Verification items for the finished model (mm, model axes). Coordinates: 2 decimals unless noted, no trailing zeros. Loops run counter-clockwise (first coordinate to the right, second up) from the corner with the lowest first, then second, coordinate; pieces in that order, holes last. Notation, with made-up numbers: (74, -35) - (131, -35) arc R30 ccw to (131, 0) - close; hole circle Ø7 at (-27, -6). An arc over 180 degrees is marked (long way). One line per item, written item: value. Start each with the question number.
(1) Gauge pin test, flat end, axial feed: P1, Ø1.5, axis at x = 122, y = 0.5, coming from the +Z side. Record the tip position at first contact, or that the pin passes through.
(2) Thickness scan on probe 1 along X at (y, z) = (0.95, 63); probe 2 along Z at (x, y) = (77, 2.3). Record the ranges inside material, lowest first. Write a range as [from, to].
(3) Section check B-B (y = 1.25). Record the boundary of the cut face in (x, z).
(4) Section check C-C (x = 91). Record the boundary of the cut face in (y, z) (3 decimals).
```python
from build123d import *

# Parameters (mm, degrees)
F0_W     = 285.75
F0_H     = 3.175
F1_DEPTH = 152.4
F3_DEPTH = 25.4


with BuildPart() as f1:
    # F0 (on Top) → F1 (new body)
    with BuildSketch(Plane.XY):
        with Locations((142.875, 1.5875)):
            Rectangle(F0_W, F0_H)
    extrude(amount=F1_DEPTH)

    # F2 (on face) → F3 (cut)
    with BuildSketch(Plane.XZ):
        Polygon((58.7375, 50.8), (142.875, 50.8), (227.0125, 50.8), (227.0125, 76.2), (227.0125, 152.4), (58.7375, 152.4), (58.7375, 76.2), align=None)
    extrude(amount=-F3_DEPTH, mode=Mode.SUBTRACT)


solid = f1.part
```
Responses:
1. P1: stops at z = 50.8
2. probe 1: x = [0, 58.74], [227.01, 285.75]
2. probe 2: z = [0, 50.8]
3. outline: (0, 0) - (285.75, 0) - (285.75, 152.4) - (227.01, 152.4) - (227.01, 50.8) - (58.74, 50.8) - (58.74, 152.4) - (0, 152.4) - close
4. outline: (0, 0) - (3.175, 0) - (3.175, 50.8) - (0, 50.8) - close
